Here's how the part is built. I have some questions about the finished solid (model axes, mm). Face numbers are marked on the shaded views. Coordinates: 2 decimals unless noted, no trailing zeros. Write each loop counter-clockwise with the first axis right and the second up, starting at its lowest first coordinate (ties: lowest second). Pieces come first, ordered by that corner, then holes. Notation, with made-up numbers: M 81,-1 L 128,-1 A23 ccw 128,34 Z; hole C 83.5,-36 d4. An arc over 180 degrees is marked long. Use one line per item in the form item = value. Start each with the question number.
1. Thinking about a two-plate mould opening in Z: for the marked faces 1 and 2, which applies, released by +Z, released by -Z, zero draft, split by the parting line, or undercut?
2. I want a section at C-C, the plane z = 5.25. List the corners of the cut face in (x, y) for me.
3. Please list where these lines run through material, in increasing order: line 1 along Y through (x, z) = (-49, 9.75); line 2 along X through (y, z) = (-29.5, 0.5); line 3 along X through (y, z) = (39.5, 5.5). Write a range as [from, to].
4. I want a section at D-D, the plane x = -21.5. List the corners of the cut face in (y, z) for me, plus the area to 3 significant figures.
5. I want a section at A-A, the plane x = -50. List the corners of the cut face in (y, z) for me, plus the area to 3 significant figures.
6. I'm going to push flat-ended pins straight in: pin 1 Ø1 at (x, z) = (7, 4) entering from -Y; pin 2 Ø1.5 at (x, z) = (-49, 5) entering from -Y; pin 3 Ø3 at (x, z) = (3.5, 8.5) entering from +Y; pin 4 Ø2 at (x, y) = (-14, -28.5) entering from +Z. Where does each tip first touch, or does it pass through?
7. I want a section at B-B, the plane y = -18.5. List the corners of the cut face in (x, z) for me, plus the area to 3 significant figures.
from build123d import *

# Parameters (mm, degrees)
SALIENTE_EXTRUIR2_DEPTH = 10


with BuildPart() as part:
    # Croquis1 → Saliente-Extruir2 (new body)
    with BuildSketch(Plane.XY):
        with BuildLine():
            Line((117.5, 85.159164705), (14.934164903, 25.942752202))
            ThreePointArc((14.934164903, 25.942752202), (-9.140901633, 23.329053884), (-27.302652317, 39.347513849))
            ThreePointArc((-27.302652317, 39.347513849), (-47.71673979, 53.763029578), (-70.412414523, 43.301270189))
            ThreePointArc((-70.412414523, 43.301270189), (-84.175170954, 0), (-70.412414523, -43.301270189))
            ThreePointArc((-70.412414523, -43.301270189), (-47.71673979, -53.763029578), (-27.302652317, -39.347513849))
            ThreePointArc((-27.302652317, -39.347513849), (-9.140901633, -23.329053884), (14.934164903, -25.942752202))
            Line((14.934164903, -25.942752202), (117.5, -85.159164705))
            ThreePointArc((117.5, -85.159164705), (137.990381057, -79.668783649), (132.5, -59.178402592))
            Line((132.5, -59.178402592), (52.5, -12.990381057))
            ThreePointArc((52.5, -12.990381057), (45, 0), (52.5, 12.990381057))
            Line((52.5, 12.990381057), (132.5, 59.178402592))
            ThreePointArc((132.5, 59.178402592), (137.990381057, 79.668783649), (117.5, 85.159164705))
        make_face()
        with BuildLine():
            ThreePointArc((-60.206207262, 36.084391824), (-71.675170954, 0), (-60.206207262, -36.084391824))
            ThreePointArc((-60.206207262, -36.084391824), (-42.783121635, -39.073720721), (-39.793792738, -21.650635095))
            ThreePointArc((-39.793792738, -21.650635095), (-46.675170954, 0), (-39.793792738, 21.650635095))
            ThreePointArc((-39.793792738, 21.650635095), (-42.783121635, 39.073720721), (-60.206207262, 36.084391824))
        make_face(mode=Mode.SUBTRACT)
    extrude(amount=SALIENTE_EXTRUIR2_DEPTH)


solid = part.part
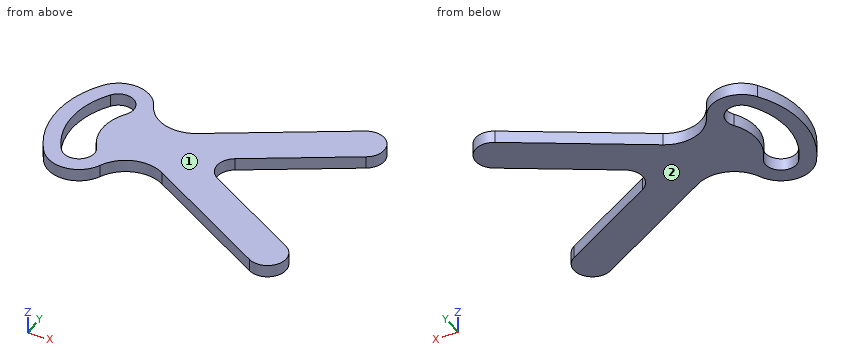
Answer list:
q1.face_1 = released by +Z
q1.face_2 = released by -Z
q2.outline = M -70.41,-43.3 A25 ccw -27.3,-39.35 A30 cw 14.93,-25.94 L 117.5,-85.16 A15 ccw 132.5,-59.18 L 52.5,-12.99 A15 cw 52.5,12.99 L 132.5,59.18 A15 ccw 117.5,85.16 L 14.93,25.94 A30 cw -27.3,39.35 A25 ccw -70.41,43.3 A75 ccw Z; hole M -60.21,-36.08 A12.5 ccw -39.79,-21.65 A37.5 cw -39.79,21.65 A12.5 ccw -60.21,36.08 A62.5 ccw Z
q3.line_1 = [-53.85, -41.33], [41.33, 53.85]
q3.line_2 = [-78.13, -64.28], [-37.52, -20], [21.1, 81.1]
q3.line_3 = [-72.93, -56.57], [-43.43, -27.37], [38.42, 98.42]
q4.outline = M -30.93,0 L 30.93,0 L 30.93,10 L -30.93,10 Z
q4.area = 619 mm²
q5.outline = M -53.87,0 L -41.37,0 L -41.37,10 L -53.87,10 Z; M 41.37,0 L 53.87,0 L 53.87,10 L 41.37,10 Z
q5.area = 250 mm²
q6.pin_1 = -22.89
q6.pin_2 = -53.87
q6.pin_3 = 22.35
q6.pin_4 = through
q7.outline = M -81.86,0 L -68.87,0 L -68.87,10 L -81.86,10 Z; M -41.79,0 L 62.04,0 L 62.04,10 L -41.79,10 Z
q7.area = 1,170 mm²
